Source: CAD feature listing. Evaluate the final solid. Frame: model axes, mm. Give positions to 0.01 mm unless a question says otherwise; leave off trailing zeros. Order: outer loops, then holes, each group sorted by start corner. A loop starts at its lowest first (then second) coordinate and runs counter-clockwise, first axis right, second up.
from build123d import *

# Parameters (mm, degrees)
F0_W     = 29
F0_H     = 13
F1_DEPTH = 1.5875
F2_R     = 6.25
F3_DEPTH = 2
F5_R     = 2.35
F6_DEPTH = 25.4


with BuildPart() as f1:
    # F0 (on Top) → F1 (new body)
    with BuildSketch(Plane.XY):
        Rectangle(F0_W, F0_H)
    extrude(amount=F1_DEPTH)

    # F5 (on face) → F6 (cut)
    with BuildSketch(Plane.XY.offset(1.5875)):
        with Locations((-12, 4)):
            Circle(F5_R)
        with Locations((-12, -4)):
            Circle(F5_R)
        with Locations((12, -4)):
            Circle(F5_R)
        with Locations((12, 4)):
            Circle(F5_R)
    extrude(amount=-F6_DEPTH, mode=Mode.SUBTRACT)


with BuildPart() as f3:
    # F2 (on Top) → F3 (new body)
    with BuildSketch(Plane.XY):
        with Locations((-62.359009, 0)):
            Circle(F2_R)
    extrude(amount=F3_DEPTH)


solid = f1.part
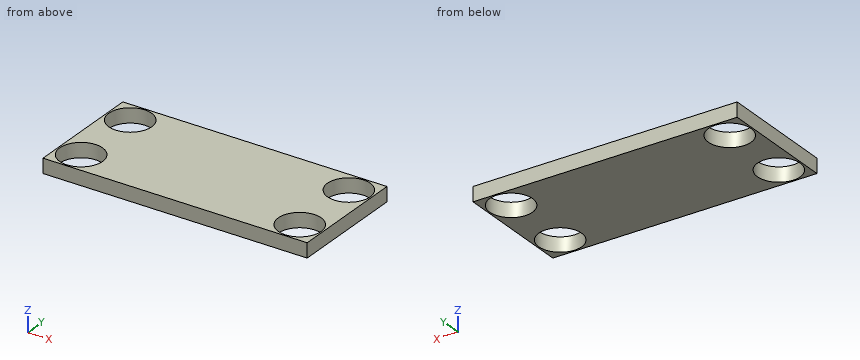
(1) Pin query (flat end, axial travel): pin 1 Ø1.5 at (x, y) = (3.5, 4) entering from -Z. Return the tip coordinate at first contact, or that it passes through.
(2) Section C-C, the plane z = 0.75. Return loops of the section in (x, y), plus the area to 3 significant figures.
(3) Section A-A, the plane x = -12. Return loops of the section in (y, z), plus the area to 4 significant figures.
(4) Line query: line 1 along Y through (x, z) = (12, 0.95); line 2 along X through (y, z) = (5.75, 0.35); line 3 along X through (y, z) = (-3.5, 1.5). Output: solid intervals per line, ascending.
(5) Section B-B, the plane y = 4. Return loops of the section in (x, z).
Checks:
1. pin 1: stops at z = 0
2. outline: (-14.5, -6.5) - (14.5, -6.5) - (14.5, 6.5) - (-14.5, 6.5) - close; hole circle Ø4.7 at (-12, -4); hole circle Ø4.7 at (-12, 4); hole circle Ø4.7 at (12, -4); hole circle Ø4.7 at (12, 4)
2. area: 308 mm2
3. outline: (-6.5, 0) - (-6.35, 0) - (-6.35, 1.59) - (-6.5, 1.59) - close; (-1.65, 0) - (1.65, 0) - (1.65, 1.59) - (-1.65, 1.59) - close; (6.35, 0) - (6.5, 0) - (6.5, 1.59) - (6.35, 1.59) - close
3. area: 5.715 mm2
4. line 1: y = -6.5 to -6.35, -1.65 to 1.65, 6.35 to 6.5
4. line 2: x = -14.5 to -13.57, -10.43 to 10.43, 13.57 to 14.5
4. line 3: x = -14.5 to -14.3, -9.7 to 9.7, 14.3 to 14.5
5. outline: (-14.5, 0) - (-14.35, 0) - (-14.35, 1.59) - (-14.5, 1.59) - close; (-9.65, 0) - (9.65, 0) - (9.65, 1.59) - (-9.65, 1.59) - close; (14.35, 0) - (14.5, 0) - (14.5, 1.59) - (14.35, 1.59) - close
